from build123d import *

# Parameters (mm, degrees)
SKETCH1_W                                        = 19.05
SKETCH1_H                                        = 57.15
BOSS_EXTRUDE1_DEPTH                              = 25.4
SKETCH2_W                                        = 17.4625
SKETCH2_H                                        = 19.05
SKETCH2_W_2                                      = 9.525
CUT_EXTRUDE1_DEPTH                               = 20.05
SKETCH9_R                                        = 3.175
CUT_EXTRUDE3_DEPTH                               = 40.6875
FILLET1_R                                        = 6.35
CBORE_FOR_1_4_SOCKET_SHOULDER_SCREW1_D           = 6.7564
CBORE_FOR_1_4_SOCKET_SHOULDER_SCREW1_CBORE_D     = 10.31748
CBORE_FOR_1_4_SOCKET_SHOULDER_SCREW1_CBORE_DEPTH = 4.7752


with BuildPart() as part:
    # Sketch1 → Boss-Extrude1 (new body)
    with BuildSketch(Plane(origin=(0, 0, 0), x_dir=(1, 0, 0), z_dir=(0, 1, 0))):
        with Locations((69.85, 0)):
            Rectangle(SKETCH1_W, SKETCH1_H)
    extrude(amount=BOSS_EXTRUDE1_DEPTH)

    # Sketch2 → Cut-Extrude1 (cut, through all)
    with BuildSketch(Plane(origin=(79.375, 0, 0), x_dir=(0, 0, -1), z_dir=(1, 0, 0))):
        with Locations((-19.84375, 15.875)):
            Rectangle(SKETCH2_W, SKETCH2_H)
        with Locations((0, 15.875)):
            Rectangle(SKETCH2_W_2, SKETCH2_H)
        with Locations((19.84375, 15.875)):
            Rectangle(SKETCH2_W, SKETCH2_H)
    extrude(amount=-CUT_EXTRUDE1_DEPTH, mode=Mode.SUBTRACT)

    # Sketch9 → Cut-Extrude3 (cut, through all)
    with BuildSketch(Plane.XY.offset(11.1125)):
        with Locations((69.85, 19.05)):
            Circle(SKETCH9_R)
    extrude(amount=-CUT_EXTRUDE3_DEPTH, mode=Mode.SUBTRACT)

    # Fillet1
    fillet1_edges = [part.edges().sort_by_distance(p)[0] for p in [
        (79.375, 25.4, 7.9375),
        (79.375, 3.175, 28.575),
        (60.325, 3.175, 28.575),
        (79.375, 25.4, -7.9375),
        (60.325, 25.4, -7.9375),
        (60.325, 25.4, 7.9375),
        (60.325, 3.175, -28.575),
        (79.375, 3.175, -28.575),
    ]]
    fillet(fillet1_edges, radius=FILLET1_R)

    # CBORE for 1/4 Socket Shoulder Screw1 (through all)
    with Locations(Plane(origin=(0, 6.35, 0), x_dir=(1, 0, 0), z_dir=(0, 1, 0))):
        with Locations((69.923370565, 18.735910675), (69.923370565, -18.735910675)):
            CounterBoreHole(CBORE_FOR_1_4_SOCKET_SHOULDER_SCREW1_D / 2, CBORE_FOR_1_4_SOCKET_SHOULDER_SCREW1_CBORE_D / 2, CBORE_FOR_1_4_SOCKET_SHOULDER_SCREW1_CBORE_DEPTH)


solid = part.part
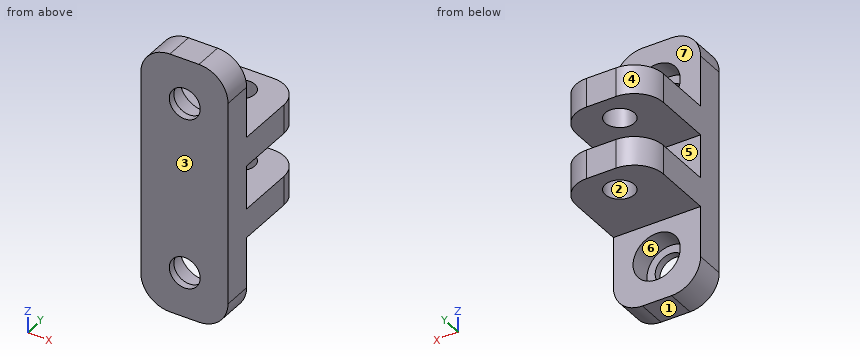
Build history of the part. All positions in model axes, mm. Face numbers are marked on the shaded views. A direction names the side the tool comes from. Round coordinates to 2 decimals unless told otherwise and drop trailing zeros. Loops run counter-clockwise (first coordinate to the right, second up) from the corner with the lowest first, then second, coordinate; pieces in that order, holes last. Notation, with made-up numbers: (80, -35.5) -> (103, -35.5) arc R30 cw to (103, -13.5) -> close; hole circle Ø2 at (40.25, 31). An arc over 180 degrees is marked (long way). Use CSV: the item, a comma, the result in double quotes. Start each with the question number.
Q1. Saw through at B-B on z = 12. Give the cut face in (x, y) (3 decimals).
Q2. Which spindle directions (+Z, -Z, +X, -X, +Y, -Y) get a long thin tool onto all of the face, cutting with end or side? Do the marked faces 5, 6 and 7. Say none if no direction does.
Q3. Mould opens along Y. For the marked faces 1, 2, 3 and 4 say: +Y half, -Y half, draft (parallel to the pull), parting line (faces both ways), or undercut.
Q4. Saw through at C-C on x = 72.25. Count the separate pieces of the cut face and the enclosed holes in it, and give its area (3 significant figures).
Q5. Saw through at A-A on y = 7. Give the cut face in (x, z) (1 decimal), and give its area (3 significant figures).
Q6. Drill centre lines: L1, parallel to Z at x = 77, y = 7.25; L2, parallel to Z at x = 74.5, y = 6.25; L3, parallel to Z at x = 73, y = 4 (3 decimals). Where is each one in solid material? Low to high.
Q7. Flat gauge pins, fed straight in: pin 1 Ø11 at (x, z) = (69.92, -18.74) entering from +Y; pin 2 Ø3 at (x, y) = (67.5, 16.5) entering from -Z; pin 3 Ø10 at (x, y) = (75.5, 17) entering from +Z. Where does each tip first touch, or does it go through?
Q8. Saw through at D-D on x = 76.5. Give the cut face in (y, z), and give its area (3 significant figures).
Solutions:
1,outline,"(60.325, 0) -> (79.375, 0) -> (79.375, 6.35) -> (60.325, 6.35) -> close"
2,face 5,"+X, -X, +Y"
2,face 6,"+Y"
2,face 7,"+Z, +X, -X, +Y"
3,face 1,"draft"
3,face 2,"undercut"
3,face 3,"-Y half"
3,face 4,"+Y half"
4,separate pieces,"5"
4,enclosed holes,"0"
4,area,"449 mm^2"
5,outline,"(60.3, -11.1) -> (79.4, -11.1) -> (79.4, -4.8) -> (60.3, -4.8) -> close; (60.3, 4.8) -> (79.4, 4.8) -> (79.4, 11.1) -> (60.3, 11.1) -> close"
5,area,"242 mm^2"
6,L1,"z = -11.11 to -4.76, 4.76 to 11.11"
6,L2,"z = -28.4 to -21.12, -16.36 to 16.36, 21.12 to 28.4"
6,L3,"z = -28.575 to -22.877, -14.595 to 14.595, 22.877 to 28.575"
7,pin 1,"stops at y = 6.35"
7,pin 2,"stops at z = -11.11"
7,pin 3,"stops at z = 11.11"
8,outline,"(0, -27.54) -> (6.35, -27.54) -> (6.35, -11.11) -> (24.36, -11.11) -> (24.36, -4.76) -> (6.35, -4.76) -> (6.35, 4.76) -> (24.36, 4.76) -> (24.36, 11.11) -> (6.35, 11.11) -> (6.35, 27.54) -> (0, 27.54) -> close"
8,area,"579 mm^2"
